Autodesk Inventor part; units mm, degrees
ref_plane "YZ Plane" through (0, 0, 0) normal (1, 0, 0) x (0, 1, 0)
ref_plane "XZ Plane" through (0, 0, 0) normal (0, 1, 0) x (-1, 0, 0)
ref_plane "XY Plane" through (0, 0, 0) normal (0, 0, 1) x (1, 0, 0)
sketch "Sketch1" plane through (0, 0, 0) normal (0, 1, 0) x (-1, 0, 0)
  line L0 (269.2628, -287.2233) -> (16.4197, -34.3803)
  circle A0 centre (270.2276, -277.5195) radius 3.3782
  line L1 (287.2233, -269.2628) -> (34.3803, -16.4197)
  line L2 (6.35, -37.5671) -> (6.35, -393.6488)
  line L3 (-6.35, -37.5671) -> (-6.35, -393.7)
  line L4 (-90.8271, -393.7) -> (-29.6915, -23.8752)
  line L5 (-101.6, -381) -> (-37.5898, 6.214)
  circle A1 centre (0, -387.35) radius 3.3782
  line L6 (37.5671, 6.35) -> (393.7, 6.35)
  line L7 (37.5671, -6.35) -> (393.6488, -6.35)
  circle A2 centre (387.35, 0) radius 3.3782
  circle A3 centre (-95.25, -387.35) radius 3.3782
  circle A4 centre (277.5195, -270.2276) radius 3.3782
  line L8 (-101.6, -381) -> (-101.6, -393.7)
  line L9 (393.7, 0) -> (393.7, 6.35)
  arc A5 (6.35, -37.5671) -> (16.4197, -34.3803) centre (0, 0) ccw
  arc A6 (34.3803, -16.4197) -> (37.5671, -6.35) centre (0, 0) ccw
  line L10 (38.1, 0) -> (38.1, 12.8556) construction
  arc A7 (37.5671, 6.35) -> (-37.5898, 6.214) centre (0, 0) ccw
  circle A8 centre (0, 0) radius 38.1 construction
  arc A9 (-6.214, 37.5898) -> (-37.5898, 6.214) centre (0, 0) ccw
  arc A10 (-29.6915, -23.8752) -> (-6.35, -37.5671) centre (0, 0) ccw
  line L11 (146.05, 0) -> (146.05, 6.35)
  line L12 (133.35, 0) -> (133.35, 6.35)
  line L13 (273.05, 6.35) -> (273.05, 0)
  line L14 (285.75, 6.35) -> (285.75, 0)
  circle A11 centre (103.1708, -94.1906) radius 3.3782
  circle A12 centre (94.1906, -103.1708) radius 3.3782
  arc A13 (393.6488, -6.35) -> (393.7, 0) centre (0, 0) ccw
  circle A14 centre (279.4, 0) radius 3.3782
  circle A15 centre (139.7, 0) radius 3.3782
  arc A16 (0, -393.7) -> (6.35, -393.6488) centre (0, 0) ccw
  arc A17 (269.2628, -287.2233) -> (287.2233, -269.2628) centre (0, 0) ccw
  circle A18 centre (202.0047, -193.0245) radius 3.3782
  circle A19 centre (193.0245, -202.0047) radius 3.3782
  circle A20 centre (0, -279.4) radius 3.3782
  line L15 (-101.6, -393.7) -> (-90.8271, -393.7)
  line L16 (-6.35, -393.7) -> (0, -393.7)
  circle A21 centre (0, -139.7) radius 3.3782
  circle A22 centre (0, 0) radius 14.2875
  circle A23 centre (-55.2746, -139.7) radius 3.3782
  circle A24 centre (-78.3684, -279.4) radius 3.3782
  line L17 (0, -285.75) -> (-6.35, -285.75)
  line L18 (-6.35, -273.05) -> (0, -273.05)
  circle A25 centre (0, -336.55) radius 3.3782
  circle A26 centre (-87.8158, -336.55) radius 3.3782
  circle A27 centre (241.5985, -234.3065) radius 3.3782
  circle A28 centre (234.3065, -241.5985) radius 3.3782
  circle A29 centre (336.55, 0) radius 3.3782
  dimension "d0" = 12.7
  dimension "d1" = 101.6
  dimension "d2" = 12.7
  dimension "d3" = 12.7
  dimension "d4" = 38.1
  dimension "d5" = 38.1
  dimension "d6" = 38.1
  dimension "d7" = 6.35
  dimension "d8" = 6.35
  dimension "d9" = 6.35
  dimension "d10" = 12.7
  dimension "d11" = 12.7
  dimension "d12" = 95.25
  dimension "d14" = 6.7564
  dimension "d15" = 6.7564
  dimension "d16" = 6.7564
  dimension "d17" = 6.35
  dimension "d18" = 6.7564
  dimension "d19" = 6.35
  dimension "d20" = 6.35
  dimension "d21" = 6.7564
  dimension "d22" = 6.7564
  dimension "d23" = 6.7564
  dimension "d25" = 6.35
  dimension "d26" = 6.7564
  dimension "d28" = 28.575
  dimension "d30" = 6.7564
  dimension "d32" = 6.7564
  dimension "d36" = 38.1
  dimension "d37" = 25.4
  dimension "d38" = 6.35
  dimension "d39" = 139.7
  dimension "d40" = 55.2746
  dimension "d41" = 139.7
  dimension "d42" = 6.35
  dimension "d43" = 6.35
  dimension "d44" = 7.3006
  dimension "d45" = 277.5195
  dimension "d46" = 270.2276
  dimension "d47" = 7.2919
  dimension "d48" = 7.2919
  dimension "d49" = 393.7
  dimension "d50" = 393.7
  dimension "d51" = 6.35
  dimension "d52" = 12.7
  dimension "d53" = 6.7564
  dimension "d54" = 6.35
  dimension "d55" = 6.7564
  dimension "d56" = 6.7564
  dimension "d57" = 393.7
  dimension "d58" = 6.35
  dimension "d60" = 6.7564
  dimension "d61" = 6.35
  dimension "d62" = 6.7564
  dimension "d63" = 6.7564
  dimension "d64" = 6.7564
  dimension "d65" = 6.7564
  dimension "d66" = 50.8
  dimension "d67" = 50.8
  dimension "d68" = 50.8
  dimension "d71" = 7.5438
  dimension "d72" = 7.5438
  dimension "d73" = 7.5438
  dimension "d74" = 7.5438
extrude "Extrusion2" add sketch "Sketch1" along normal blind 6.35
sketch "Sketch6" plane through (0, 6.35, 0) normal (0, 1, 0) x (1, 0, 0)
  line L0 (-16.4197, 34.3803) -> (-269.2628, 287.2233)
  line L1 (-287.2233, 269.2628) -> (-34.3803, 16.4197)
  line L2 (-393.7, -6.35) -> (-37.5671, -6.35)
  line L3 (101.6, 381) -> (101.6, 393.7)
  arc A0 (0, 393.7) -> (-6.35, 393.6488) centre (0, 0) ccw
  line L4 (0, 0) -> (-287.2233, 287.2233) construction
  circle A1 centre (0, 0) radius 14.2875
  line L5 (-37.5671, 6.35) -> (-393.6488, 6.35)
  line L6 (6.35, 37.5671) -> (6.35, 393.7)
  circle A2 centre (-107.7631, 107.7631) radius 3.3782
  circle A3 centre (-143.6841, 143.6841) radius 3.3782
  line L7 (-146.05, 464.3998) -> (-146.05, -90.5947) construction
  circle A4 centre (-203.2, 0) radius 3.3782
  circle A5 centre (-152.4, 0) radius 3.3782
  line L8 (-146.05, -6.35) -> (-146.05, 6.35)
  line L9 (-209.55, 6.35) -> (-209.55, -6.35)
  line L10 (-139.194, 157.1545) -> (-157.1545, 139.194)
  line L11 (-112.2532, 94.2927) -> (-94.2927, 112.2532)
  line L12 (-209.55, 6.35) -> (-157.1545, 139.194)
  line L13 (-112.2532, 94.2927) -> (-146.05, 6.35)
  line L14 (-183.3522, 72.772) -> (-129.1516, 50.3213)
  dimension "d115" = 6.7564
  dimension "d117" = 6.7564
  dimension "d118" = 247.65
  dimension "d122" = 152.4
  dimension "d123" = 203.2
  dimension "d124" = 6.7564
  dimension "d126" = 152.4
  dimension "d127" = 203.2
  dimension "d129" = 6.35
  dimension "d130" = 6.35
  dimension "d131" = 6.35
  dimension "d132" = 6.35
extrude "Extrusion8" cut sketch "Sketch6" against normal blind 25.4 contours A2 | A3 | A4 | A5
sketch "Sketch8" plane through (0, 6.35, 0) normal (0, 1, 0) x (1, 0, 0)
  circle A0 centre (0, 0) radius 14.2875
  arc A1 (0, 393.7) -> (-6.35, 393.6488) centre (0, 0) ccw
  circle A2 centre (0, 0) radius 9.5
  dimension "d135" = 19
extrude "Extrusion9" add sketch "Sketch8" against normal blind 6.35
sketch "Sketch9" plane through (0, 6.35, 0) normal (0, 1, 0) x (1, 0, 0)
  circle A0 centre (95.25, 365.2157) radius 3.3782
extrude "Extrusion10" cut sketch "Sketch9" against normal blind 25.4
equation "\"d71\" = d74"
equation "\"d72\" = d73"
properties part number "Bearing Mount v1" material "Aluminum 6061"
The listing builds one solid part. Answer for the finished solid, in the listing's coordinates (mm). A direction names the side the tool comes from. Coordinates: 2 decimals unless noted, no trailing zeros. Write each loop counter-clockwise with the first axis right and the second up, starting at its lowest first coordinate (ties: lowest second). Pieces come first, ordered by that corner, then holes. Notation, with made-up numbers: M 11,49.25 L 24,49.25 A22 cw 24,60.25 Z; hole C 4,51 d7. An arc over 180 degrees is marked long. Put each result on its own line as item: value. Start each with the question number.
1. A cutting plane is placed at B-B on x = -293. Write down the section's boundary in (y, z).
2. A cutting plane is placed at C-C on y = 3.75. Count the separate pieces of the cut face and the enclosed holes in it, then the cut area to 3 significant figures.
3. Flat-ended cylindrical pins translate along their axes: P1, Ø1, axis at x = 27.5, y = 3.5, coming from the +Z side; P2, Ø3, axis at x = -201, y = 4, coming from the +Z side; P3, Ø3, axis at y = 3, z = -169, coming from the -X side. Find the tip coordinate at first contact, or state that the pin passes through.
4. Consider line 1 (Z direction, x = 0, y = 2.25); line 2 (Z direction, x = -137.5, y = 1); line 3 (X direction, y = 5.75, z = -192.5). Determine where each line is inside the solid, lowest interval first. Write a range as from..to.
5. For a pull along X with two mould halves and no side action, classify faces 4 (the flat face through (-144.61, 3.13, -162.57)), 5 (the cylindrical face through (-278.514, 3.131, -278.262)), 6 (the flat face through (70.043, 3.131, -190.103)) as pulls with the +X half, pulls with the -X half, needs draft (parallel to the pull), parting line crosses it, or undercut.
6. Which of the six approach directions +Z, -Z, +X, -X, +Y, -Y give full straight-line access (tool end or side, diameter ignored) to faces 1 (the flat face through (60.687, 3.131, -211.376)), 2 (the cylindrical face through (4.38, 3.22, 8.43)), 3 (the flat face through (-162.57, 3.13, -144.61))?
7. A cutting plane is placed at A-A on z = -261.5. Write down the section's boundary in (x, y), then the cut area to 3 significant figures.
Resolved:
1. outline: M 0,-6.35 L 6.35,-6.35 L 6.35,6.35 L 0,6.35 Z
2. separate pieces: 1
2. enclosed holes: 26
2. area: 26,300 mm2
3. P1: stops at z = 26.88
3. P2: stops at z = 6.35
3. P3: stops at x = -188.46
4. line 1: z = -393.7..-390.73, -383.97..-339.93, -333.17..-282.78, -276.02..-143.08, -136.32..-9.5, 9.5..38.1
4. line 2: z = -155.46..-119.54, -6.35..-2.56, 2.56..6.35
4. line 3: x = -210.46..-205.34, -198.67..-174.54, -6.35..6.35, 57.57..70.44
5. face 4: undercut
5. face 5: pulls with the -X half
5. face 6: pulls with the +X half
6. face 1: -Z, +Y, -Y
6. face 2: +Y, -Y
6. face 3: -X, +Y, -Y
7. outline: M -279.46,0 L -243.54,0 L -243.54,6.35 L -279.46,6.35 Z; M -6.35,0 L 6.35,0 L 6.35,6.35 L -6.35,6.35 Z; M 68.97,0 L 81.85,0 L 81.85,6.35 L 68.97,6.35 Z
7. area: 390 mm2
